Verification items for this drawing (mm, ordinates from the low corner). Round coordinates to 2 decimals unless told otherwise and drop trailing zeros. Loops run counter-clockwise (first coordinate to the right, second up) from the corner with the lowest first, then second, coordinate; pieces in that order, holes last. Notation, with made-up numbers: (58.5, 53) -> (77.5, 53) arc R21 cw to (77.5, 84) -> close; hole circle Ø6 at (-29, 2). An arc over 180 degrees is marked (long way). Use a Markdown table: item, result. Add a question column.
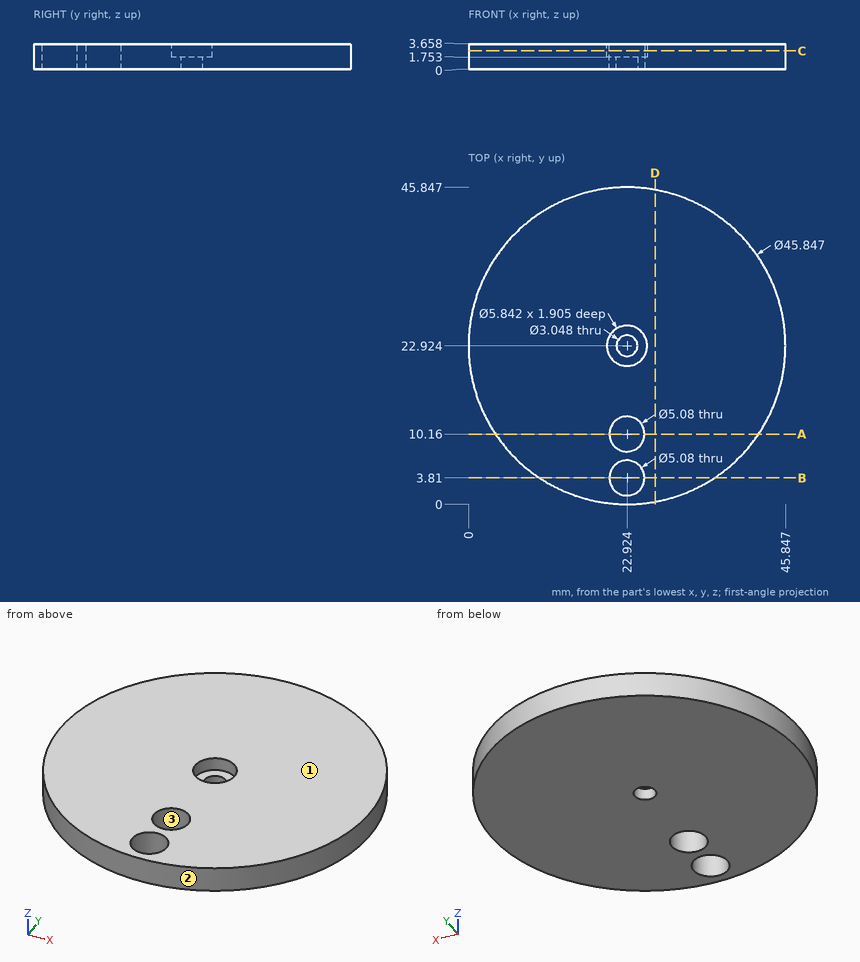
1) Thickness scan on line 1 (Y direction, x = 10.5, z = 2.2); line 2 (Y direction, x = 16, z = 0.45) (1 decimal); line 3 (X direction, y = 26, z = 2.35). Record the ranges inside material, lowest first.
2) Sectioned sample at A-A on y = 10.16. Enter the section's corners in (x, z) (1 decimal), then the cut area to 3 significant figures.
3) Sectioned sample at C-C on z = 2.65. Enter the section's corners in (x, y) (1 decimal), then the cut area to 3 significant figures.
4) Release check for a two-part mould opening along Y. For the marked faces 1, 2 and 3 record: released by +Y, released by -Y, zero draft, split by the parting line, or undercut.
5) Sectioned sample at D-D on x = 27. Enter the section's corners in (y, z) (1 decimal).
6) Go/stop test with flat-tipped pins: pin 1 (1.5 mm diameter, centred on x = 26, z = 1.5, fed in from +Y); pin 2 (1 mm diameter, centred on y = 8, z = 1.5, fed in from +X); pin 3 (1 mm diameter, centred on x = 16, z = 2.5, fed in from +Y). Record where each tip stops, or that it passes through.
7) Sectioned sample at B-B on y = 3.81. Enter the section's corners in (x, z).
Geometry results:
| question | item | result |
|---|---|---|
| 1 | line 1 | 3.66 to 42.19 |
| 1 | line 2 | 1.1 to 44.8 |
| 1 | line 3 | 0.21 to 45.64 |
| 2 | outline | (3.9, 0) -> (20.4, 0) -> (20.4, 3.7) -> (3.9, 3.7) -> close; (25.5, 0) -> (42, 0) -> (42, 3.7) -> (25.5, 3.7) -> close |
| 2 | area | 121 mm^2 |
| 3 | outline | circle Ø45.8 at (22.9, 22.9); hole circle Ø5.8 at (22.9, 22.9); hole circle Ø5.1 at (22.9, 3.8); hole circle Ø5.1 at (22.9, 10.2) |
| 3 | area | 1,580 mm^2 |
| 4 | face 1 | zero draft |
| 4 | face 2 | split by the parting line |
| 4 | face 3 | undercut |
| 5 | outline | (0.4, 0) -> (45.5, 0) -> (45.5, 3.7) -> (0.4, 3.7) -> close |
| 6 | pin 1 | y = 45.73 |
| 6 | pin 2 | x = 40.74 |
| 6 | pin 3 | y = 44.93 |
| 7 | outline | (10.27, 0) -> (20.38, 0) -> (20.38, 3.66) -> (10.27, 3.66) -> close; (25.46, 0) -> (35.58, 0) -> (35.58, 3.66) -> (25.46, 3.66) -> close |
